Job drawing, mm, ordinate dimensions from the low corner. One solid piece. A direction names the side the tool comes from. Round coordinates to 2 decimals unless told otherwise and drop trailing zeros. Write each loop counter-clockwise with the first axis right and the second up, starting at its lowest first coordinate (ties: lowest second). Pieces come first, ordered by that corner, then holes.
1) Saw through at C-C (y = 14). Write the cut outline in (x, z), plus the area to 3 significant figures.
2) Pull direction Y, two halves, no side cores. Call the marked faces 3, 4, 5 and 6: +Y half, -Y half, draft (parallel to the pull), parting line (faces both ways), or undercut.
3) Saw through at A-A (z = 1.75). Write the cut outline in (x, y).
4) Saw through at B-B (x = 12.5). Write the cut outline in (y, z).
5) Which spindle directions (+Z, -Z, +X, -X, +Y, -Y) get a long thin tool onto all of the face, cutting with end or side? Do the marked faces 1 and 2. Say none if no direction does.
6) Wall check: probe 1 along Y at (x, z) = (10.75, 0.5); probe 2 along Z at (x, y) = (1.5, 13.5). Give the ranges that are in metal, low to high.
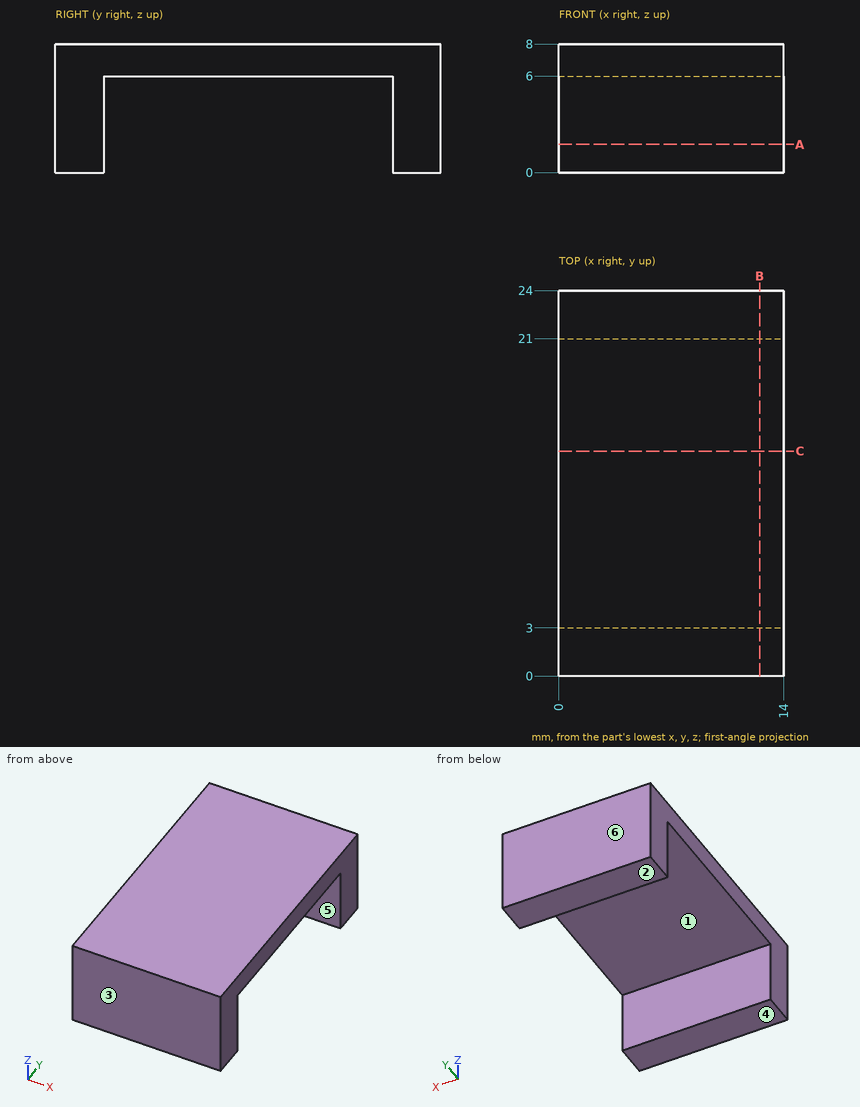
Evaluation:
1. outline: (0, 6) - (14, 6) - (14, 8) - (0, 8) - close
1. area: 28.0 mm2
2. face 3: -Y half
2. face 4: draft
2. face 5: undercut
2. face 6: +Y half
3. outline: (0, 0) - (14, 0) - (14, 3) - (0, 3) - close; (0, 21) - (14, 21) - (14, 24) - (0, 24) - close
4. outline: (0, 0) - (3, 0) - (3, 6) - (21, 6) - (21, 0) - (24, 0) - (24, 8) - (0, 8) - close
5. face 1: -Z, +X, -X
5. face 2: -Z, +X, -X, +Y, -Y
6. probe 1: y = 0 to 3, 21 to 24
6. probe 2: z = 6 to 8
